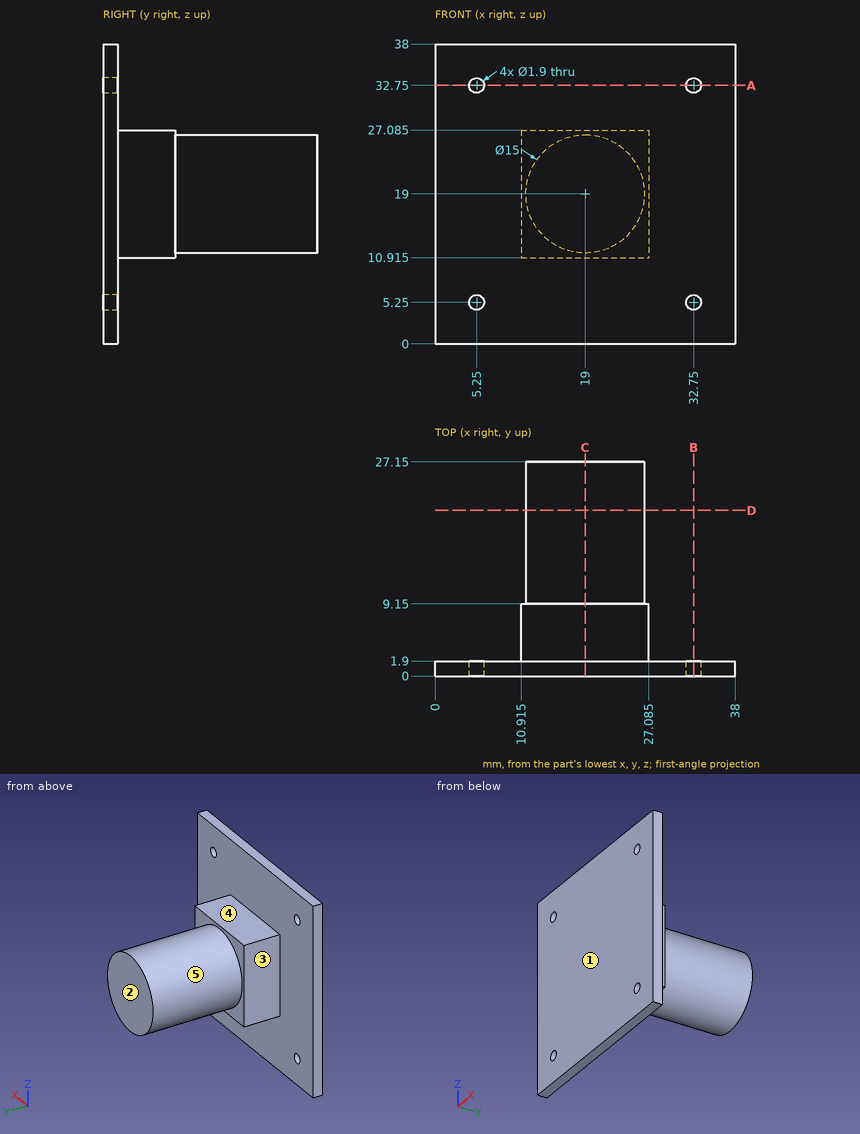
Design review of the part shown in the three views and the two pictorial views. Dimensions are in mm from the part's minimum x, y and z. A direction names the side the tool comes from. Round coordinates to 2 decimals unless told otherwise and drop trailing zeros. Write each loop counter-clockwise with the first axis right and the second up, starting at its lowest first coordinate (ties: lowest second). Pieces come first, ordered by that corner, then holes.
1) Take a section at C-C on x = 19. Give the boundary of the cut face in (y, z) (3 decimals), then the cut area to 3 significant figures.
Answer below:
outline: (0, 0) - (1.9, 0) - (1.9, 10.915) - (9.15, 10.915) - (9.15, 11.5) - (27.15, 11.5) - (27.15, 26.5) - (9.15, 26.5) - (9.15, 27.085) - (1.9, 27.085) - (1.9, 38) - (0, 38) - close
area: 459 mm2
2) Take a section at D-D on y = 21. Give the boundary of the cut face in (x, z), then the cut area to 3 significant figures.
Answer below:
outline: circle Ø15 at (19, 19)
area: 177 mm2
3) Take a section at B-B on x = 32.75. Give the boundary of the cut face in (y, z), then the cut area to 3 significant figures.
Answer below:
outline: (0, 0) - (1.9, 0) - (1.9, 4.3) - (0, 4.3) - close; (0, 6.2) - (1.9, 6.2) - (1.9, 31.8) - (0, 31.8) - close; (0, 33.7) - (1.9, 33.7) - (1.9, 38) - (0, 38) - close
area: 65.0 mm2
4) Take a section at A-A on z = 32.75. Give the boundary of the cut face in (x, y).
Answer below:
outline: (0, 0) - (4.3, 0) - (4.3, 1.9) - (0, 1.9) - close; (6.2, 0) - (31.8, 0) - (31.8, 1.9) - (6.2, 1.9) - close; (33.7, 0) - (38, 0) - (38, 1.9) - (33.7, 1.9) - close
5) For line 1 along X through (y, z) = (1.45, 32.75); line 2 along Y through (x, z) = (3, 11.5), list the stretches that pass through material, from the lowest coordinate up.
Answer below:
line 1: x = 0 to 4.3, 6.2 to 31.8, 33.7 to 38
line 2: y = 0 to 1.9
6) Insertion check: pin 1 Ø3.5 at (y, z) = (5, 18) entering from +X (3 decimals); pin 2 Ø8 at (x, y) = (16.5, 4) entering from -Z; pin 3 Ø2 at (x, y) = (15.5, 5) entering from +Z (3 decimals); pin 4 Ø2 at (x, z) = (33.5, 17) entering from +Y. Each pin has a flat end and moves straight along its axis. Give the tip position at first contact, or say it passes through.
Answer below:
pin 1: stops at x = 27.085
pin 2: stops at z = 0
pin 3: stops at z = 27.085
pin 4: stops at y = 1.9
7) Mouldability with a two-part tool opening along Y and no side actions: class the marked faces 1, 2 and 3 as +Y half, -Y half, draft (parallel to the pull), parting line (faces both ways), or undercut.
Answer below:
face 1: -Y half
face 2: +Y half
face 3: draft
8) Machinability: for the marked faces 4 and 5, which of the approach directions +Z, -Z, +X, -X, +Y, -Y give a long, thin tool a straight path to every point of the face, cutting with its end or side? Answer none if there is none.
Answer below:
face 4: +Z, +X, -X, +Y
face 5: +Y
